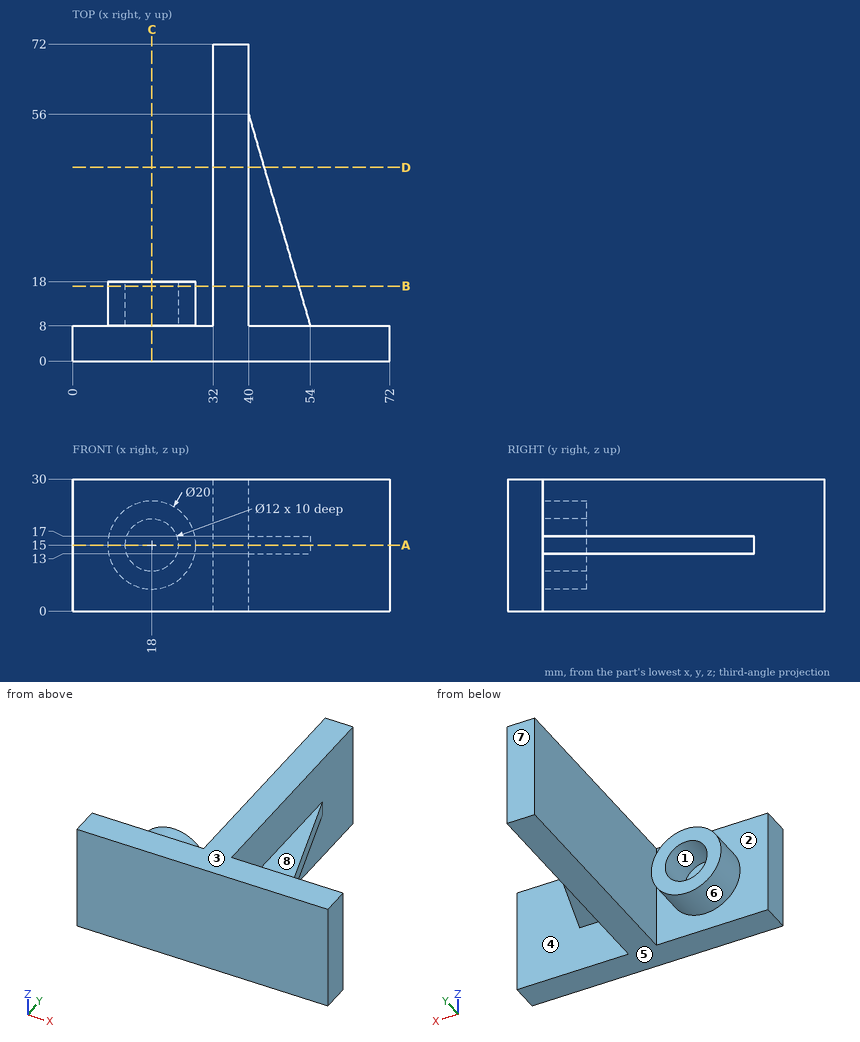
Answer from the drawing. Dimensions are ordinates in mm from the lowest x, y and z of the part. A direction names the side the tool comes from. Give positions to 0.01 mm unless a question says otherwise; leave off trailing zeros. Order: outer loops, then holes, each group sorted by start corner. A loop starts at its lowest first (then second) coordinate and runs counter-clockwise, first axis right, second up.
Item 1: The part is cut by section D-D, the plane y = 44. Give the vertices of the cut face in (x, z), and give its area (3 significant figures).
From the geometry:
outline: (32, 0) - (40, 0) - (40, 13) - (43.5, 13) - (43.5, 17) - (40, 17) - (40, 30) - (32, 30) - close
area: 254 mm2
Item 2: Find the intervals of material crossed by probe 1 along Z at (x, y) = (18, 15); probe 2 along X at (y, z) = (16.25, 15); probe 3 along X at (y, z) = (12, 18), in increasing order.
From the geometry:
probe 1: z = 5 to 9, 21 to 25
probe 2: x = 8 to 12, 24 to 28, 32 to 51.59
probe 3: x = 8.46 to 12.8, 23.2 to 27.54, 32 to 40
Item 3: Which of the six approach directions +Z, -Z, +X, -X, +Y, -Y give full straight-line access (tool end or side, diameter ignored) to the marked faces 4, 5, 6, 7 and 8?
From the geometry:
face 4: +X, +Y
face 5: -Z, +X, -X, +Y, -Y
face 6: +Y
face 7: +Z, -Z, +X, -X, +Y
face 8: +Z, +X, +Y
Item 4: Given pin 1 Ø12 at (x, z) = (14, 5) entering from +Y; pin 2 Ø5 at (x, y) = (49.5, 16) entering from -Z; pin 3 Ø6 at (x, z) = (18.5, 12.5) entering from +Y; pin 4 Ø15.5 at (x, y) = (45, 21) entering from -Z, each flat-ended and moving along its own axis, determine where each tip first touches the part or whether it passes through.
From the geometry:
pin 1: stops at y = 18
pin 2: stops at z = 13
pin 3: stops at y = 8
pin 4: stops at z = 0
Item 5: The part is cut by section B-B, the plane y = 17. Give the vertices of the cut face in (x, z) (3 decimals), and give its area (3 significant figures).
From the geometry:
outline: circle Ø20 at (18, 15); (32, 0) - (40, 0) - (40, 13) - (51.375, 13) - (51.375, 17) - (40, 17) - (40, 30) - (32, 30) - close; hole circle Ø12 at (18, 15)
area: 487 mm2
Item 6: For a pull along Z with two mould halves and no side action, classify the marked faces 1, 2 and 3 as pulls with the +Z half, pulls with the -Z half, needs draft (parallel to the pull), parting line crosses it, or undercut.
From the geometry:
face 1: undercut
face 2: needs draft
face 3: pulls with the +Z half
Item 7: The part is cut by section A-A, the plane z = 15. Give the vertices of the cut face in (x, y), and give its area (3 significant figures).
From the geometry:
outline: (0, 0) - (72, 0) - (72, 8) - (54, 8) - (40, 56) - (40, 72) - (32, 72) - (32, 8) - (28, 8) - (28, 18) - (24, 18) - (24, 8) - (12, 8) - (12, 18) - (8, 18) - (8, 8) - (0, 8) - close
area: 1,500 mm2
Item 8: The part is cut by section C-C, the plane x = 18. Give the vertices of the cut face in (y, z), and give its area (3 significant figures).
From the geometry:
outline: (0, 0) - (8, 0) - (8, 5) - (18, 5) - (18, 9) - (8, 9) - (8, 21) - (18, 21) - (18, 25) - (8, 25) - (8, 30) - (0, 30) - close
area: 320 mm2
